```python
from build123d import *

# Parameters (mm, degrees)
SKETCH_1_R          = 20
SKETCH_1_R_2        = 7
EXTRUDE_1_DEPTH     = 20
SKETCH_2_R          = 20
EXTRUDE_2_DEPTH     = 10
SKETCH_3_R          = 3
CUT_EXTRUDE_1_DEPTH = 10
SKETCH_4_R          = 3.5
CUT_EXTRUDE_2_DEPTH = 25


with BuildPart() as part:
    # 草图1 → 凸台-拉伸1 (new body)
    with BuildSketch(Plane.XY):
        Circle(SKETCH_1_R)
        Circle(SKETCH_1_R_2, mode=Mode.SUBTRACT)
    extrude(amount=EXTRUDE_1_DEPTH)

    # 草图2 → 凸台-拉伸2 (add)
    with BuildSketch(Plane.XY.offset(20)):
        Circle(SKETCH_2_R)
    extrude(amount=EXTRUDE_2_DEPTH)

    # 草图3 → 切除-拉伸1 (cut)
    with BuildSketch(Plane.XY.offset(30)):
        Circle(SKETCH_3_R)
    extrude(amount=-CUT_EXTRUDE_1_DEPTH, mode=Mode.SUBTRACT)

    # 草图4 → 切除-拉伸2 (cut)
    with BuildSketch(Plane(origin=(0, 0, 0), x_dir=(-1, 0, 0), z_dir=(0, 0, -1))):
        with Locations((0, 12)):
            Circle(SKETCH_4_R)
    extrude(amount=-CUT_EXTRUDE_2_DEPTH, mode=Mode.SUBTRACT)


solid = part.part
```
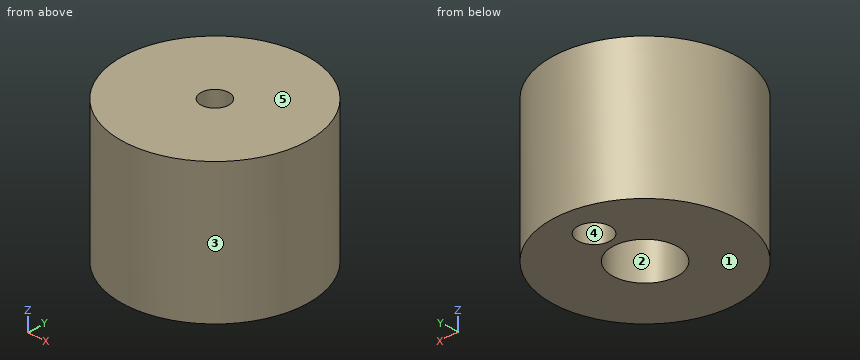
Work out the finished part from the listing and answer in its coordinate system (mm). Face numbers are marked on the shaded views. A direction names the side the tool comes from. Round coordinates to 2 decimals unless told otherwise and drop trailing zeros. Write each loop counter-clockwise with the first axis right and the second up, starting at its lowest first coordinate (ties: lowest second). Pieces come first, ordered by that corner, then holes.
1) A cutting plane is placed at D-D on y = 12. Determine the outline of the cut face in (x, z).
2) A cutting plane is placed at B-B on x = 0. Determine the outline of the cut face in (y, z), and give its area (3 significant figures).
3) Which of the six approach directions +Z, -Z, +X, -X, +Y, -Y give full straight-line access (tool end or side, diameter ignored) to the marked faces 4 and 5?
4) A cutting plane is placed at A-A on y = 0. Determine the outline of the cut face in (x, z), and give its area (3 significant figures).
5) Consider probe 1 along Y at (x, z) = (0, 24.5); probe 2 along Y at (x, z) = (0, 8.5); probe 3 along X at (y, z) = (-5.5, 13.25). Determine where each line is inside the solid, lowest interval first.
6) A cutting plane is placed at C-C on z = 14. Determine the outline of the cut face in (x, y), and give its area (3 significant figures).
7) Determine the mould class of the marked faces 1, 2 and 3 for opening direction Y: pulls with the +Y half, pulls with the -Y half, needs draft (parallel to the pull), parting line crosses it, or undercut.
8) Flat-ended cylindrical pins translate along their axes: P1, Ø10, axis at x = -0.5, z = 15, coming from the -Y side; P2, Ø12, axis at y = -14.5, z = 5, coming from the -X side; P3, Ø5, axis at y = -5, z = 10, coming from the -X side. Find the tip coordinate at first contact, or state that the pin passes through.
Entries:
1. outline: (-16, 0) - (-3.5, 0) - (-3.5, 25) - (3.5, 25) - (3.5, 0) - (16, 0) - (16, 30) - (-16, 30) - close
2. outline: (-20, 0) - (-7, 0) - (-7, 20) - (-3, 20) - (-3, 30) - (-20, 30) - close; (3, 20) - (7, 20) - (7, 0) - (8.5, 0) - (8.5, 25) - (15.5, 25) - (15.5, 0) - (20, 0) - (20, 30) - (3, 30) - close
2. area: 685 mm2
3. face 4: -Z
3. face 5: +Z, +X, -X, +Y, -Y
4. outline: (-20, 0) - (-7, 0) - (-7, 20) - (-3, 20) - (-3, 30) - (-20, 30) - close; (3, 20) - (7, 20) - (7, 0) - (20, 0) - (20, 30) - (3, 30) - close
4. area: 860 mm2
5. probe 1: y = -20 to -3, 3 to 8.5, 15.5 to 20
5. probe 2: y = -20 to -7, 7 to 8.5, 15.5 to 20
5. probe 3: x = -19.23 to -4.33, 4.33 to 19.23
6. outline: circle Ø40 at (0, 0); hole circle Ø14 at (0, 0); hole circle Ø7 at (0, 12)
6. area: 1,060 mm2
7. face 1: needs draft
7. face 2: undercut
7. face 3: parting line crosses it
8. P1: stops at y = -20
8. P2: stops at x = -18.1
8. P3: stops at x = -19.84
